Verification items for the finished model (mm, model axes). A direction names the side the tool comes from. Give positions to 0.01 mm unless a question says otherwise; leave off trailing zeros. Loops run counter-clockwise (first coordinate to the right, second up) from the corner with the lowest first, then second, coordinate; pieces in that order, holes last. Notation, with made-up numbers: (-18.5, 65) - (10.5, 65) arc R29 ccw to (10.5, 91) - close; hole circle Ø6 at (66.25, 40.5). An arc over 180 degrees is marked (long way). One line per item, written item: value. Start each with the question number.
1. Sectioned sample at A-A (z = 12). Record the cut outline in (x, y), plus the area to 3 significant figures.
2. Access from +Z, -Z, +X, -X, +Y, -Y to the whole of each face (thin tool, end or side, straight path). Record for faces 1 (the flat face through (-5, -3, 8.825)), 2 (the flat face through (6.35, 0, 12)), 3 (the cylindrical face through (4.143, -1.305, 16.939)), 4 (the cylindrical face through (4.143, -1.305, 25.525)).
3. Scan lines: L1, parallel to Y at x = 0, z = 18.5; L2, parallel to Z at x = 0.75, y = -5.75; L3, parallel to Y at x = 0.5, z = 10.75. Record each from-to range of solid material in increasing order. Write a range as [from, to].
4. Gauge pin test, flat ends, axial feed: pin 1 (6 mm diameter, centred on x = 2, y = 1, fed in from -Z); pin 2 (1 mm diameter, centred on x = -3.5, y = 2, fed in from +Z); pin 3 (4 mm diameter, centred on x = -2, z = 16, fed in from -Y); pin 4 (1 mm diameter, centred on x = -4.5, z = 14.5, fed in from -Y). Record the tip position at first contact, or that the pin passes through.
5. Sectioned sample at C-C (z = 25.75). Record the cut outline in (x, y).
from build123d import *

# Parameters (mm, degrees)
SKETCH2_OUTSIDE_W  = 26.768
SKETCH2_OUTSIDE_H  = 26.768
CUT_EXTRUDE1_DEPTH = 31.938714767


with BuildPart() as part:
    # Sketch1 → Revolve1 (revolve)
    with BuildSketch(Plane(origin=(0, 0, 0), x_dir=(0, 0, -1), z_dir=(1, 0, 0)), mode=Mode.PRIVATE) as revolve1_sk:
        Polygon((-12.809985226, 2.3876), (-28.426098562, 2.3876), (-28.426098562, 2.7686), (-26.336268377, 4.3434), (-24.736068377, 4.3434), (-24.292315867, 5.5626), (-18.413231404, 5.5626), (-17.969478894, 4.3434), (-15.937478894, 4.3434), (-15.937478894, 6.096), (-15.012994499, 8.636), (-9.749963289, 8.636), (-8.825478894, 6.096), (-8.825478894, 5.1562), (0, 4.539062397), (0, 2.5781), (-12.7, 2.5781), align=None)
    revolve(revolve1_sk.sketch.rotate(Axis((0, 0, -2.001994087), (0, 0, -1)), 90), axis=Axis((0, 0, -2.001994087), (0, 0, -1)))

    # Sketch2 outside → Cut-Extrude1 (cut, through all)
    with BuildSketch(Plane.XY):
        Rectangle(SKETCH2_OUTSIDE_W, SKETCH2_OUTSIDE_H)
        Polygon((0, 7.332348419), (-6.35, 3.666174209), (-6.35, -3.666174209), (0, -7.332348419), (6.35, -3.666174209), (6.35, 3.666174209), align=None, mode=Mode.SUBTRACT)
    extrude(amount=CUT_EXTRUDE1_DEPTH, mode=Mode.SUBTRACT)


solid = part.part
Results are:
1. outline: (-6.35, -3.67) - (0, -7.33) - (6.35, -3.67) - (6.35, 3.67) - (0, 7.33) - (-6.35, 3.67) - close; hole circle Ø5.16 at (0, 0)
1. area: 119 mm^2
2. face 1: -Z
2. face 2: +Z, -Z, +X, +Y, -Y
2. face 3: none
2. face 4: +Z
3. L1: y = [-5.56, -2.39], [2.39, 5.56]
3. L2: z = [8.83, 15.94]
3. L3: y = [-7.04, -2.53], [2.53, 7.04]
4. pin 1: stops at z = 0
4. pin 2: stops at z = 27.41
4. pin 3: stops at y = -7.3
4. pin 4: stops at y = -5.02
5. outline: circle Ø8.69 at (0, 0); hole circle Ø4.78 at (0, 0)
